from build123d import *

# Parameters (mm, degrees)
BOSS_EXTRUDE1_DEPTH                                  = 10
CUT_EXTRUDE1_REACH                                   = 76.458
SKETCH2_R                                            = 7
CSK_FOR_M8_FLAT_HEAD_MACHINE_SCREW1_D                = 7
CSK_FOR_M8_FLAT_HEAD_MACHINE_SCREW1_CSINK_D          = 8
CSK_FOR_M8_FLAT_HEAD_MACHINE_SCREW1_CSINK_ANGLE      = 90
M4X0_7_TAPPED_HOLE1_REACH                            = 76.458
M4X0_7_TAPPED_HOLE1_BORE_R                           = 2
CUT_EXTRUDE2_REACH                                   = 78.446
SKETCH8_R                                            = 2.5
CUT_EXTRUDE3_REACH                                   = 76.458
CUT_EXTRUDE3_END_RADIUS                              = 2.5
SKETCH9_R                                            = 1.25
TAP_DRILL_FOR_M3_5X0_6_TAP1_D                        = 2.9
TAP_DRILL_FOR_M3_5X0_6_TAP1_DEPTH                    = 9
TAP_DRILL_FOR_M3_5X0_6_TAP1_TIP                      = 0.871247898
CUT_EXTRUDE4_REACH                                   = 76.458
CUT_EXTRUDE4_END_RADIUS                              = 7
SKETCH14_R                                           = 1.6
CBORE_FOR_M4_CROSS_RECESS_PAN_HEAD_SCREW_D           = 2.5
CBORE_FOR_M4_CROSS_RECESS_PAN_HEAD_SCREW_CBORE_D     = 4
CBORE_FOR_M4_CROSS_RECESS_PAN_HEAD_SCREW_CBORE_DEPTH = 30
CUT_EXTRUDE5_DEPTH                                   = 2
SKETCH18_R                                           = 6
CUT_EXTRUDE6_DEPTH                                   = 1
CHAMFER1_SIZE                                        = 0.5


with BuildPart() as part:
    # Sketch1 → Boss-Extrude1 (new, symmetric)
    with BuildSketch(Plane.XY):
        Polygon((0, 0), (0, 24), (-12, 62), (-40, 62), (-40, 30), (-21, 30), (-21, 0), align=None)
    extrude(amount=BOSS_EXTRUDE1_DEPTH, both=True)

    # Sketch2 → Cut-Extrude1 (cut, up to next)
    with BuildSketch(Plane(origin=(0, 62, 0), x_dir=(1, 0, 0), z_dir=(0, 1, 0)), mode=Mode.PRIVATE) as cut_extrude1_sk1:
        with Locations(Location((-30, 0, 0), (0, 0, 270))):
            Circle(SKETCH2_R)
    cut_extrude1_tool1 = extrude(cut_extrude1_sk1.sketch, amount=-CUT_EXTRUDE1_REACH, mode=Mode.PRIVATE) & part.part
    add(cut_extrude1_tool1.solids().sort_by_distance((-30, 62, 0))[0], mode=Mode.SUBTRACT)

    # CSK for M8 Flat Head Machine Screw1 (through all)
    with Locations(Plane(origin=(0, 0, 0), x_dir=(0, 0, -1), z_dir=(1, 0, 0))):
        with Locations((0, 10)):
            CounterSinkHole(CSK_FOR_M8_FLAT_HEAD_MACHINE_SCREW1_D / 2, CSK_FOR_M8_FLAT_HEAD_MACHINE_SCREW1_CSINK_D / 2, counter_sink_angle=CSK_FOR_M8_FLAT_HEAD_MACHINE_SCREW1_CSINK_ANGLE)

    # M4x0.7 Tapped Hole1 bore → M4x0.7 Tapped Hole1 (cut, up to next)
    with BuildSketch(Plane(origin=(0, 0, 0), x_dir=(-1, 0, 0), z_dir=(0, -1, 0)), mode=Mode.PRIVATE) as m4x0_7_tapped_hole1_sk1:
        with Locations((8, 0)):
            Circle(M4X0_7_TAPPED_HOLE1_BORE_R)
    m4x0_7_tapped_hole1_tool1 = extrude(m4x0_7_tapped_hole1_sk1.sketch, amount=-M4X0_7_TAPPED_HOLE1_REACH, mode=Mode.PRIVATE) & part.part
    # M4x0.7 Tapped Hole1 bore → M4x0.7 Tapped Hole1 (cut, up to next)
    with BuildSketch(Plane(origin=(0, 0, 0), x_dir=(-1, 0, 0), z_dir=(0, -1, 0)), mode=Mode.PRIVATE) as m4x0_7_tapped_hole1_sk2:
        with Locations((16, 0)):
            Circle(M4X0_7_TAPPED_HOLE1_BORE_R)
    m4x0_7_tapped_hole1_tool2 = extrude(m4x0_7_tapped_hole1_sk2.sketch, amount=-M4X0_7_TAPPED_HOLE1_REACH, mode=Mode.PRIVATE) & part.part
    add(m4x0_7_tapped_hole1_tool1.solids().sort_by_distance((-8, 0, 0))[0], mode=Mode.SUBTRACT)
    add(m4x0_7_tapped_hole1_tool2.solids().sort_by_distance((-16, 0, 0))[0], mode=Mode.SUBTRACT)

    # Sketch8 → Cut-Extrude2 (cut, up to next)
    with BuildSketch(Plane.XY.offset(10), mode=Mode.PRIVATE) as cut_extrude2_sk1:
        with Locations((-8, 20)):
            Circle(SKETCH8_R)
    cut_extrude2_tool1 = extrude(cut_extrude2_sk1.sketch, amount=-CUT_EXTRUDE2_REACH, mode=Mode.PRIVATE) & part.part
    add(cut_extrude2_tool1.solids().sort_by_distance((-8, 20, 10))[0], mode=Mode.SUBTRACT)

    # Cut-Extrude3: up to this cylinder (the profile starts outside it)
    cut_extrude3_end = Plane(origin=(-8, 20, 0), z_dir=(0, 0, 1)) * Cylinder(CUT_EXTRUDE3_END_RADIUS, 158.916, mode=Mode.PRIVATE)
    # Sketch9 → Cut-Extrude3 (cut, up to the surface)
    with BuildSketch(Plane.XZ, mode=Mode.PRIVATE) as cut_extrude3_sk1:
        with Locations(Location((-8, 0, 0), (0, 0, 270))):
            Circle(SKETCH9_R)
    cut_extrude3_tool1 = extrude(cut_extrude3_sk1.sketch, amount=-CUT_EXTRUDE3_REACH, mode=Mode.PRIVATE) - cut_extrude3_end
    add(cut_extrude3_tool1.solids().sort_by_distance((-8, 0, 0))[0], mode=Mode.SUBTRACT)

    # Tap Drill for M3.5x0.6 Tap1
    with Locations(Plane(origin=(0, 62, 0), x_dir=(1, 0, 0), z_dir=(0, 1, 0))):
        with Locations((-37, 7), (-16, 7), (-16, -7), (-37, -7)):
            Hole(TAP_DRILL_FOR_M3_5X0_6_TAP1_D / 2, depth=TAP_DRILL_FOR_M3_5X0_6_TAP1_DEPTH)
            with Locations((0, 0, -(TAP_DRILL_FOR_M3_5X0_6_TAP1_DEPTH + TAP_DRILL_FOR_M3_5X0_6_TAP1_TIP / 2))):  # 118° drill point
                Cone(0, TAP_DRILL_FOR_M3_5X0_6_TAP1_D / 2, TAP_DRILL_FOR_M3_5X0_6_TAP1_TIP, mode=Mode.SUBTRACT)

    # Cut-Extrude4: up to this cylinder (the profile starts outside it)
    cut_extrude4_end = Plane(origin=(-30, 45, 0), z_dir=(0, 1, 0)) * Cylinder(CUT_EXTRUDE4_END_RADIUS, 167.916, mode=Mode.PRIVATE)
    # Sketch14 → Cut-Extrude4 (cut, up to the surface)
    with BuildSketch(Plane.ZY.offset(40), mode=Mode.PRIVATE) as cut_extrude4_sk1:
        with Locations(Location((-3, 45, 0), (0, 0, 270))):
            Circle(SKETCH14_R)
    cut_extrude4_tool1 = extrude(cut_extrude4_sk1.sketch, amount=-CUT_EXTRUDE4_REACH, mode=Mode.PRIVATE) - cut_extrude4_end
    add(cut_extrude4_tool1.solids().sort_by_distance((-40, 45, -3))[0], mode=Mode.SUBTRACT)
    # Sketch14 → Cut-Extrude4 (cut, up to the surface)
    with BuildSketch(Plane.ZY.offset(40), mode=Mode.PRIVATE) as cut_extrude4_sk2:
        with Locations(Location((3, 45, 0), (0, 0, 270))):
            Circle(SKETCH14_R)
    cut_extrude4_tool2 = extrude(cut_extrude4_sk2.sketch, amount=-CUT_EXTRUDE4_REACH, mode=Mode.PRIVATE) - cut_extrude4_end
    add(cut_extrude4_tool2.solids().sort_by_distance((-40, 45, 3))[0], mode=Mode.SUBTRACT)

    # CBORE for M4 Cross Recess Pan Head Screw1 (through all)
    with Locations(Plane(origin=(0, 62, 0), x_dir=(1, 0, 0), z_dir=(0, 1, 0))):
        with Locations((-16, 0)):
            CounterBoreHole(CBORE_FOR_M4_CROSS_RECESS_PAN_HEAD_SCREW_D / 2, CBORE_FOR_M4_CROSS_RECESS_PAN_HEAD_SCREW_CBORE_D / 2, CBORE_FOR_M4_CROSS_RECESS_PAN_HEAD_SCREW_CBORE_DEPTH)

    # Sketch17 → Cut-Extrude5 (cut)
    with BuildSketch(Plane(origin=(0, 62, 0), x_dir=(1, 0, 0), z_dir=(0, 1, 0))):
        with BuildLine():
            Line((-16.110062598, 1.99696926), (-16.110062598, 2))
            Line((-16.110062598, 2), (-23.291796068, 2))
            ThreePointArc((-23.291796068, 2), (-23.073333142, 1.010587075), (-23, 0))
            ThreePointArc((-23, 0), (-23.073333142, -1.010587075), (-23.291796068, -2))
            Line((-23.291796068, -2), (-16.110062598, -2))
            Line((-16.110062598, -2), (-16.110062598, -1.99696926))
            ThreePointArc((-16.110062598, -1.99696926), (-18, 0), (-16.110062598, 1.99696926))
        make_face()
    extrude(amount=-CUT_EXTRUDE5_DEPTH, mode=Mode.SUBTRACT)

    # Sketch18 → Cut-Extrude6 (cut)
    with BuildSketch(Plane(origin=(0, 0, 0), x_dir=(0, 0, -1), z_dir=(1, 0, 0))):
        with Locations((0, 10)):
            Circle(SKETCH18_R)
    extrude(amount=-CUT_EXTRUDE6_DEPTH, mode=Mode.SUBTRACT)

    # Chamfer1
    chamfer1_edges = [part.edges().sort_by_distance(p)[0] for p in [
        (-21, 10, -3.5),
    ]]
    chamfer(chamfer1_edges, length=CHAMFER1_SIZE)


solid = part.part
Read the model definition and answer for the solid it produces. Units are mm, in the model's axes. A direction names the side the tool comes from. Round coordinates to 2 decimals unless told otherwise and drop trailing zeros. Write each loop counter-clockwise with the first axis right and the second up, starting at its lowest first coordinate (ties: lowest second). Pieces come first, ordered by that corner, then holes. Notation, with made-up numbers: (-9, -18.5) - (17, -18.5) arc R13 ccw to (17, -11.5) - close; hole circle Ø5 at (-31.75, -37). An arc over 180 degrees is marked (long way). One line per question, with ' | ' between items. Start each with the question number.
1. For faces 4 (the face through (-8.76, 15.52, 0.99)), 5 (the face through (-38.19, 45.35, -4.56)), 6 (the face through (-17.38, 57.44, -7.44)), determine the directions among +Z, -Z, +X, -X, +Y, -Y from which every point of the face is accessible in a straight line to the end or side of a thin tool.
2. Section A-A (x = -30) is taken. Determine the outline of the cut face in (y, z), and give its area (3 significant figures).
3. For a pull along X with two mould halves and no side action, classify faces 1 (the face through (-40, 46, 0)), 2 (the face through (-17.339, 57.437, 7.555)), 3 (the face through (-0.493, 4.143, 1.301)) as +X half, -X half, draft (parallel to the pull), parting line (faces both ways), or undercut.
4. Section C-C (z = 0) is taken. Give the number of separate pieces and of enclosed holes in the cut face, and give its area (3 significant figures).
5. Find the intervals of material crossed by probe 1 along Z at (x, y) = (-16, 58); probe 2 along Z at (x, y) = (-38.8, 45); probe 3 along X at (y, z) = (39, -0.75), in increasing order. Write a range as [from, to].
6. Section D-D (x = -8) is taken. Determine the outline of the cut face in (y, z), and give its area (3 significant figures).
7. Section B-B (y = 44.5) is taken. Determine the outline of the cut face in (x, z), and give its area (3 significant figures).
8. Each of these flat-tipped pins is pushed along its axis until it touches: pin 1 (5.5 mm diameter, centred on x = -27, z = -1.5, fed in from -Y); pin 2 (4.5 mm diameter, centred on x = -37, z = 7, fed in from -Y); pin 3 (2 mm diameter, centred on y = 31, z = 5, fed in from +X). Where does it stop, or does it pass through?
Filled in:
1) face 4: -Y | face 5: -X | face 6: +Y
2) outline: (30, -10) - (62, -10) - (62, -7) - (30, -7) - close; (30, 7) - (62, 7) - (62, 10) - (30, 10) - close | area: 192 mm²
3) face 1: -X half | face 2: undercut | face 3: draft
4) separate pieces: 6 | enclosed holes: 0 | area: 824 mm²
5) probe 1: [-10, -8.45], [-5.55, -2], [2, 5.55], [8.45, 10] | probe 2: [-10, -4.6], [-1.4, 1.4], [4.6, 10] | probe 3: [-40, -36.96], [-23.04, -17.85], [-14.15, -4.74]
6) outline: (0, -10) - (17.5, -10) - (17.5, -1.25) - (13.27, -1.25) arc R3.5 cw to (7.13, -2) - (0, -2) - close; (0, 2) - (7.13, 2) arc R3.5 cw to (13.27, 1.25) - (17.5, 1.25) - (17.5, 10) - (0, 10) - close; (22.5, -10) - (49.33, -10) - (49.33, 10) - (22.5, 10) - close | area: 811 mm²
7) outline: (-40, -10) - (-6.47, -10) - (-6.47, 10) - (-40, 10) - (-40, 4.52) - (-35.35, 4.52) arc R7 cw (long way) to (-35.35, -4.52) - (-40, -4.52) - close; (-40, -1.48) - (-36.84, -1.48) arc R7 cw to (-36.84, 1.48) - (-40, 1.48) - close; hole circle Ø4 at (-16, 0) | area: 481 mm²
8) pin 1: through | pin 2: y = 30 | pin 3: x = -1.89
